Drawing for the job (mm, zero at the part's lowest x, y, z). A direction names the side the tool comes from. Coordinates: 2 decimals unless noted, no trailing zeros. Loops run counter-clockwise (first coordinate to the right, second up) from the corner with the lowest first, then second, coordinate; pieces in that order, holes last. Notation, with made-up numbers: (0, 24.25) - (22, 24.25) arc R16 ccw to (22, 29.25) - close; hole circle Ø10 at (45.25, 88). An arc over 180 degrees is marked (long way). One line per item, written item: value.
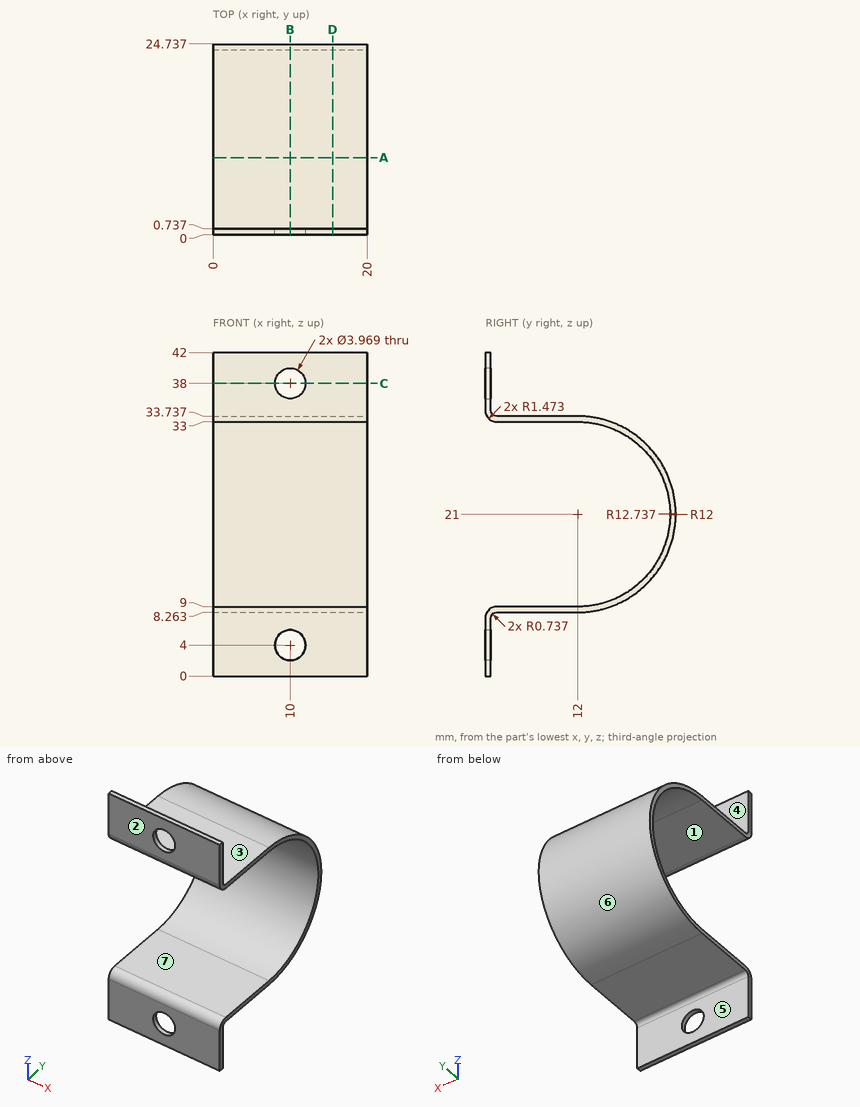
Item 1: Cut at B-B, the plane x = 10. Write the cut outline in (y, z) (1 decimal).
Check result:
outline: (0, 0) - (0.7, 0) - (0.7, 2) - (0, 2) - close; (0, 6) - (0.7, 6) - (0.7, 7.5) arc R0.7 cw to (1.5, 8.3) - (12, 8.3) arc R12.7 ccw to (12, 33.7) - (1.5, 33.7) arc R0.7 cw to (0.7, 34.5) - (0.7, 36) - (0, 36) - (0, 34.5) arc R1.5 ccw to (1.5, 33) - (12, 33) arc R12 cw to (12, 9) - (1.5, 9) arc R1.5 ccw to (0, 7.5) - close; (0, 40) - (0.7, 40) - (0.7, 42) - (0, 42) - close
Item 2: Probe probe 1 along Z at (x, y) = (8, 4); probe 2 along X at (y, z) = (0.25, 38) (1 decimal); probe 3 along Z at (x, y) = (1.75, 16.5) (1 decimal). List the from-to ranges inside material, lowest first. Write a range as from..to.
Check result:
probe 1: z = 8.26..9, 33..33.74
probe 2: x = 0..8, 12..20
probe 3: z = 9.1..9.9, 32.1..32.9
Item 3: Cut at A-A, the plane y = 10. Write the cut outline in (x, z).
Check result:
outline: (0, 8.26) - (20, 8.26) - (20, 9) - (0, 9) - close; (0, 33) - (20, 33) - (20, 33.74) - (0, 33.74) - close
Item 4: Cut at D-D, the plane x = 15.5. Write the cut outline in (y, z).
Check result:
outline: (0, 0) - (0.74, 0) - (0.74, 7.53) arc R0.74 cw to (1.47, 8.26) - (12, 8.26) arc R12.74 ccw to (12, 33.74) - (1.47, 33.74) arc R0.74 cw to (0.74, 34.47) - (0.74, 42) - (0, 42) - (0, 34.47) arc R1.47 ccw to (1.47, 33) - (12, 33) arc R12 cw to (12, 9) - (1.47, 9) arc R1.47 ccw to (0, 7.53) - close
Item 5: Pull direction Z, two halves, no side cores. Call the marked faces 1, 2 and 3: released by +Z, released by -Z, zero draft, split by the parting line, or undercut.
Check result:
face 1: undercut
face 2: zero draft
face 3: released by +Z
Item 6: Tool access for the marked faces 4, 5, 6 and 7: list every direction of +Z, -Z, +X, -X, +Y, -Y with a clear straight run to the whole face (end or side of a thin tool).
Check result:
face 4: +Z, +X, -X, +Y
face 5: -Z, +X, -X, +Y
face 6: +X, -X, +Y
face 7: +X, -X, -Y
Item 7: Drop flat-ended pins along their axis: P1, Ø5.5, axis at x = 14, y = 4, coming from the +Z side; P2, Ø3, axis at x = 16, y = 5.5, coming from the +Z side; P3, Ø3, axis at x = 2, z = 27.5, coming from the -Y side (1 decimal). Give the stop position or say it passes through.
Check result:
P1: stops at z = 33.77
P2: stops at z = 33.74
P3: stops at y = 20.9
Item 8: Cut at C-C, the plane z = 38. Write the cut outline in (x, y) (1 decimal), then the cut area to 3 significant figures.
Check result:
outline: (0, 0) - (8, 0) - (8, 0.7) - (0, 0.7) - close; (12, 0) - (20, 0) - (20, 0.7) - (12, 0.7) - close
area: 11.8 mm^2
